```python
from build123d import *

# Parameters (mm, degrees)
SKETCH1_W           = 100
SKETCH1_H           = 25
BOSS_EXTRUDE1_DEPTH = 25
CUT_EXTRUDE1_DEPTH  = 48
SKETCH3_W           = 4
SKETCH3_H           = 18
CUT_EXTRUDE2_DEPTH  = 104.832798286
SKETCH4_R           = 2.122448424
CUT_EXTRUDE3_DEPTH  = 62.23724357
SKETCH5_W           = 100
SKETCH5_H           = 3
CUT_EXTRUDE4_DEPTH  = 62.23724357


with BuildPart() as part:
    # Sketch1 → Boss-Extrude1 (new body)
    with BuildSketch(Plane(origin=(0, 0, 0), x_dir=(1, 0, 0), z_dir=(0, 1, 0))):
        Rectangle(SKETCH1_W, SKETCH1_H)
    extrude(amount=BOSS_EXTRUDE1_DEPTH)

    # Sketch2 → Cut-Extrude1 (cut)
    with BuildSketch(Plane.XY.offset(12.5)):
        with BuildLine():
            Line((-19.5, 19), (-19.5, 0))
            Line((-19.5, 0), (-24.5, 0))
            Line((-24.5, 0), (-24.5, 19))
            ThreePointArc((-24.5, 19), (-22, 21.5), (-19.5, 19))
        make_face()
        with BuildLine():
            Line((-46.5, 19), (-46.5, 0))
            Line((-46.5, 0), (-41.5, 0))
            Line((-41.5, 0), (-41.5, 19))
            ThreePointArc((-41.5, 19), (-44, 21.5), (-46.5, 19))
        make_face()
        with BuildLine():
            Line((2.5, 19), (2.5, 0))
            Line((2.5, 0), (-2.5, 0))
            Line((-2.5, 0), (-2.5, 19))
            ThreePointArc((-2.5, 19), (0, 21.5), (2.5, 19))
        make_face()
        with BuildLine():
            Line((24.5, 19), (24.5, 0))
            Line((24.5, 0), (19.5, 0))
            Line((19.5, 0), (19.5, 19))
            ThreePointArc((19.5, 19), (22, 21.5), (24.5, 19))
        make_face()
        with BuildLine():
            Line((46.5, 19), (46.5, 0))
            Line((46.5, 0), (41.5, 0))
            Line((41.5, 0), (41.5, 19))
            ThreePointArc((41.5, 19), (44, 21.5), (46.5, 19))
        make_face()
    extrude(amount=-CUT_EXTRUDE1_DEPTH, mode=Mode.SUBTRACT)

    # Sketch3 → Cut-Extrude2 (cut, through all)
    with BuildSketch(Plane.ZY.offset(50)):
        with Locations((0, 9)):
            Rectangle(SKETCH3_W, SKETCH3_H)
    extrude(amount=-CUT_EXTRUDE2_DEPTH, mode=Mode.SUBTRACT)

    # Sketch4 → Cut-Extrude3 (cut, through all)
    with BuildSketch(Plane.XY.offset(12.5)):
        with Locations((-33, 10)):
            Circle(SKETCH4_R)
        with Locations(Location((33, 10, 0), (0, 0, 270))):
            Circle(SKETCH4_R)
    extrude(amount=-CUT_EXTRUDE3_DEPTH, mode=Mode.SUBTRACT)

    # Sketch5 → Cut-Extrude4 (cut, through all)
    with BuildSketch(Plane.XY.offset(12.5)):
        with Locations((0, 1.5)):
            Rectangle(SKETCH5_W, SKETCH5_H)
    extrude(amount=-CUT_EXTRUDE4_DEPTH, mode=Mode.SUBTRACT)


solid = part.part
```
Geometry: final body of the model. Coordinates: model frame, mm. A direction names the side the tool comes from. Coordinates: 2 decimals unless noted, no trailing zeros. Loops run counter-clockwise (first coordinate to the right, second up) from the corner with the lowest first, then second, coordinate; pieces in that order, holes last. Notation, with made-up numbers: M -32,55.5 L 6,55.5 A27 ccw 6,85.5 Z; hole C 89.25,24 d5. An arc over 180 degrees is marked long. Put each result on its own line as item: value.
(1) Material intervals for probe 1 along X at (y, z) = (13.25, 10); probe 2 along Z at (x, y) = (37.5, 6.5); probe 3 along Y at (x, z) = (-33, -9.5), sorted ascending.
Answer sheet:
probe 1: x = -50 to -46.5, -41.5 to -24.5, -19.5 to -2.5, 2.5 to 19.5, 24.5 to 41.5, 46.5 to 50
probe 2: z = -12.5 to -2, 2 to 12.5
probe 3: y = 3 to 7.88, 12.12 to 25
(2) Cut plane A-A on x = -33. Return the cut outline in (y, z).
Answer sheet:
outline: M 3,-12.5 L 7.88,-12.5 L 7.88,-2 L 3,-2 Z; M 3,2 L 7.88,2 L 7.88,12.5 L 3,12.5 Z; M 12.12,-12.5 L 25,-12.5 L 25,12.5 L 12.12,12.5 L 12.12,2 L 18,2 L 18,-2 L 12.12,-2 Z
(3) First-contact query: pin 1 (1.8 mm diameter, centred on x = -47.5, z = -1, fed in from -Y). Flat tip, straight axial feed; report the tip coordinate or a pass-through.
Answer sheet:
pin 1: stops at y = 18
(4) Access query for faces 1 (the face through (-35.12, 10.09, 7.32)), 2 (the face through (-19.5, 11, 3)), 3 (the face through (11, 10, 2)). Directions: +Z, -Z, +X, -X, +Y, -Y. A direction counts if a zero-diameter tool reaches every point of the face in a straight line with its end or side. Return the directions, or none.
Answer sheet:
face 1: +Z, -Z
face 2: +Z, -Z, -Y
face 3: +X, -X, -Y
(5) Cut plane D-D on x = -14.5. Return the cut outline in (y, z).
Answer sheet:
outline: M 3,-12.5 L 25,-12.5 L 25,12.5 L 3,12.5 L 3,2 L 18,2 L 18,-2 L 3,-2 Z
(6) Cut plane B-B on z = -4.5. Return the cut outline in (x, y), then the cut area to 3 significant figures.
Answer sheet:
outline: M -50,3 L -46.5,3 L -46.5,19 A2.5 cw -41.5,19 L -41.5,3 L -24.5,3 L -24.5,19 A2.5 cw -19.5,19 L -19.5,3 L -2.5,3 L -2.5,19 A2.5 cw 2.5,19 L 2.5,3 L 19.5,3 L 19.5,19 A2.5 cw 24.5,19 L 24.5,3 L 41.5,3 L 41.5,19 A2.5 cw 46.5,19 L 46.5,3 L 50,3 L 50,25 L -50,25 Z; hole C -33,10 d4.24; hole C 33,10 d4.24
area: 1,720 mm^2
(7) Cut plane C-C on y = 10. State how many separate pieces and enclosed holes the cut face has, then the cut area to 3 significant figures.
Answer sheet:
separate pieces: 16
enclosed holes: 0
area: 1,400 mm^2
(8) Draft query along Y for faces 4 (the face through (24.5, 11, 3)), 5 (the face through (-33, 18, 0)), 6 (the face through (-35.12, 10.09, -7.18)). Return one class per face: pulls with the +Y half, pulls with the -Y half, needs draft (parallel to the pull), parting line crosses it, or undercut.
Answer sheet:
face 4: needs draft
face 5: pulls with the -Y half
face 6: undercut
